```python
from build123d import *

# Parameters (mm, degrees)
SKETCH_1_W          = 60.2
SKETCH_1_H          = 30
EXTRUDE_1_DEPTH     = 2
SKETCH_2_R          = 1.35
CUT_EXTRUDE_1_DEPTH = 3
SKETCH_3_R          = 2.35
SKETCH_3_R_2        = 1.35
EXTRUDE_2_DEPTH     = 5
SKETCH_4_W          = 3
SKETCH_4_H          = 30
EXTRUDE_3_DEPTH     = 6
SKETCH_5_R          = 1.5
CUT_EXTRUDE_2_DEPTH = 37


with BuildPart() as part:
    # 草图1 → 凸台-拉伸1 (new body)
    with BuildSketch(Plane(origin=(0, 0, 0), x_dir=(1, 0, 0), z_dir=(0, 1, 0))):
        Rectangle(SKETCH_1_W, SKETCH_1_H)
    extrude(amount=EXTRUDE_1_DEPTH)

    # 草图2 → 切除-拉伸1 (cut, through all)
    with BuildSketch(Plane(origin=(0, 2, 0), x_dir=(1, 0, 0), z_dir=(0, 1, 0))):
        with Locations((-27.65, 10.65)):
            Circle(SKETCH_2_R)
        with Locations((-27.65, -10.65)):
            Circle(SKETCH_2_R)
        with Locations((27.65, -10.65)):
            Circle(SKETCH_2_R)
        with Locations((27.65, 10.65)):
            Circle(SKETCH_2_R)
    extrude(amount=-CUT_EXTRUDE_1_DEPTH, mode=Mode.SUBTRACT)

    # 草图3 → 凸台-拉伸2 (add)
    with BuildSketch(Plane(origin=(0, 2, 0), x_dir=(1, 0, 0), z_dir=(0, 1, 0))):
        with Locations((-27.65, 10.65)):
            Circle(SKETCH_3_R)
        with Locations((-27.65, 10.65)):
            Circle(SKETCH_3_R_2, mode=Mode.SUBTRACT)
        with Locations((27.65, 10.65)):
            Circle(SKETCH_3_R)
        with Locations((27.65, 10.65)):
            Circle(SKETCH_3_R_2, mode=Mode.SUBTRACT)
        with Locations((27.65, -10.65)):
            Circle(SKETCH_3_R)
        with Locations((27.65, -10.65)):
            Circle(SKETCH_3_R_2, mode=Mode.SUBTRACT)
        with Locations((-27.65, -10.65)):
            Circle(SKETCH_3_R)
        with Locations((-27.65, -10.65)):
            Circle(SKETCH_3_R_2, mode=Mode.SUBTRACT)
    extrude(amount=EXTRUDE_2_DEPTH)

    # 草图4 → 凸台-拉伸3 (add)
    with BuildSketch(Plane.XZ):
        with Locations((4.4, 0)):
            Rectangle(SKETCH_4_W, SKETCH_4_H)
        with Locations((-4.4, 0)):
            Rectangle(SKETCH_4_W, SKETCH_4_H)
    extrude(amount=EXTRUDE_3_DEPTH)

    # 草图5 → 切除-拉伸2 (cut, through all)
    with BuildSketch(Plane.ZY.offset(5.9)):
        with Locations((-7, -3.75)):
            Circle(SKETCH_5_R)
        with Locations((7.35, -3.75)):
            Circle(SKETCH_5_R)
    extrude(amount=-CUT_EXTRUDE_2_DEPTH, mode=Mode.SUBTRACT)


solid = part.part
```
Geometry: final body of the model. Coordinates: model frame, mm. A direction names the side the tool comes from. Coordinates: 2 decimals unless noted, no trailing zeros. Write each loop counter-clockwise with the first axis right and the second up, starting at its lowest first coordinate (ties: lowest second). Pieces come first, ordered by that corner, then holes. Notation, with made-up numbers: M -1,78 L 58,78 A17 cw 58,100 Z; hole C 27,9 d11. An arc over 180 degrees is marked long. Use CSV: the item, a comma, the result in double quotes. Start each with the question number.
1. Mould query, pull axis X, two halves, no side actions, for faces 1 (the face through (18, 0, 0)), 2 (the face through (-29.38, 4.46, -12.24)), 3 (the face through (30.1, 1, 0)). Classes: pulls with the +X half, pulls with the -X half, needs draft (parallel to the pull), parting line crosses it, or undercut.
2. Cut plane D-D on y = -3.75. Return the cut outline in (x, z), plus the area to 3 significant figures.
3. Cut plane C-C on x = -27.65. Return the cut outline in (y, z).
4. Ray query, probe 1 along X at (y, z) = (3.8, 10.65); probe 2 along X at (y, z) = (1.3, 10.65); probe 3 along Z at (x, y) = (27.65, 1). Return the intervals inside material, ascending.
5. Cut plane A-A on y = 3.5. Return the cut outline in (x, z).
6. Reachability of faces 4 (the face through (-26, 7, 11)), 5 (the face through (2.9, -3, 0)), 6 (the face through (-5.9, -3, 0)), 7 (the face through (29.8, 4.5, 11.6)) from +Z, -Z, +X, -X, +Y, -Y: full face, straight path, thin tool, end or side. Return the list, or none.
7. Cut plane B-B on z = -7. Return the cut outline in (x, y).
8. First-contact query: P1, Ø8, axis at x = 13.5, z = -8.5, coming from the -Y side; P2, Ø10, axis at x = 22, z = 3, coming from the +Y side; P3, Ø5, axis at y = -3.75, z = 7.35, coming from the +X side. Flat tips, straight axial feed; report the tip coordinate or a pass-through.
Entries:
1,face 1,"needs draft"
1,face 2,"undercut"
1,face 3,"pulls with the +X half"
2,outline,"M -5.9,-15 L -2.9,-15 L -2.9,-8.5 L -5.9,-8.5 Z; M -5.9,-5.5 L -2.9,-5.5 L -2.9,5.85 L -5.9,5.85 Z; M -5.9,8.85 L -2.9,8.85 L -2.9,15 L -5.9,15 Z; M 2.9,-15 L 5.9,-15 L 5.9,-8.5 L 2.9,-8.5 Z; M 2.9,-5.5 L 5.9,-5.5 L 5.9,5.85 L 2.9,5.85 Z; M 2.9,8.85 L 5.9,8.85 L 5.9,15 L 2.9,15 Z"
2,area,"144 mm²"
3,outline,"M 0,-15 L 2,-15 L 2,-13 L 7,-13 L 7,-12 L 0,-12 Z; M 0,-9.3 L 7,-9.3 L 7,-8.3 L 2,-8.3 L 2,8.3 L 7,8.3 L 7,9.3 L 0,9.3 Z; M 0,12 L 7,12 L 7,13 L 2,13 L 2,15 L 0,15 Z"
4,probe 1,"-30 to -29, -26.3 to -25.3, 25.3 to 26.3, 29 to 30"
4,probe 2,"-30.1 to -29, -26.3 to 26.3, 29 to 30.1"
4,probe 3,"-15 to -12, -9.3 to 9.3, 12 to 15"
5,outline,"C -27.65,-10.65 d4.7; C -27.65,10.65 d4.7; C 27.65,-10.65 d4.7; C 27.65,10.65 d4.7; hole C -27.65,-10.65 d2.7; hole C -27.65,10.65 d2.7; hole C 27.65,-10.65 d2.7; hole C 27.65,10.65 d2.7"
6,face 4,"+Z, -Z, +X, -X, +Y"
6,face 5,"+Z, -Z, -Y"
6,face 6,"+Z, -Z, -X, -Y"
6,face 7,"+Y"
7,outline,"M -30.1,0 L -5.9,0 L -5.9,-2.25 L -2.9,-2.25 L -2.9,0 L 2.9,0 L 2.9,-2.25 L 5.9,-2.25 L 5.9,0 L 30.1,0 L 30.1,2 L -30.1,2 Z; M -5.9,-6 L -2.9,-6 L -2.9,-5.25 L -5.9,-5.25 Z; M 2.9,-6 L 5.9,-6 L 5.9,-5.25 L 2.9,-5.25 Z"
8,P1,"y = 0"
8,P2,"y = 2"
8,P3,"x = 5.9"
